Geometry check sheet. Reference: the model listing, model coordinates, mm. A direction names the side the tool comes from. Give positions to 0.01 mm unless a question says otherwise; leave off trailing zeros. Loops run counter-clockwise (first coordinate to the right, second up) from the corner with the lowest first, then second, coordinate; pieces in that order, holes last. Notation, with made-up numbers: (62, 76) -> (94, 76) arc R25 ccw to (94, 114) -> close; hole circle Ø10 at (59, 4.25). An arc over 180 degrees is marked (long way). One line per item, written item: value. Start each with the question number.
(1) Tool access check on faces 4 (the face through (5, -2, 10)), 5 (the face through (-1.73, -7.81, 6.96)). Record the directions out of +Z, -Z, +X, -X, +Y, -Y that give a thin tool (end or side, any length) a straight path to the whole face; none if there is none.
(2) Sectioned sample at A-A, the plane y = 0. Record the cut outline in (x, z).
(3) Draft check along Y on faces 1 (the face through (-14.985, 0.66, 1.986)), 2 (the face through (4.006, 1.262, 4.944)), 3 (the face through (6, -6, 4)). Enter one of: pulls with the +Y half, pulls with the -Y half, needs draft (parallel to the pull), parting line crosses it, or undercut.
(4) Scan lines: line 1 along Y through (x, z) = (-0.25, 8.75); line 2 along Z through (x, y) = (-10.5, 4.75); line 3 along X through (y, z) = (2, 2.5). Record each from-to range of solid material in increasing order. Write a range as from..to.
(5) Gauge pin test, flat ends, axial feed: pin 1 Ø5 at (x, z) = (-9, 9) entering from -Y; pin 2 Ø4 at (x, z) = (-9, 8) entering from -Y; pin 3 Ø9.5 at (x, y) = (0, 0) entering from -Z. Record the tip position at first contact, or that the pin passes through.
(6) Sectioned sample at C-C, the plane z = 2.5. Record the cut outline in (x, y).
from build123d import *

# Parameters (mm, degrees)
CYLINDER_R        = 15
CYLINDER_DEPTH    = 4
CYLINDER002_R     = 8
CYLINDER002_DEPTH = 10
CYLINDER003_R     = 4.2
CYLINDER003_DEPTH = 10
CHAMFER_SIZE      = 1
CHAMFER001_SIZE   = 1


with BuildPart() as part:
    # Cylinder → Cylinder (join)
    with BuildSketch(Plane.XY):
        Circle(CYLINDER_R)
    extrude(amount=CYLINDER_DEPTH)

    # Cylinder002 → Cylinder002 (join)
    with BuildSketch(Plane.XY):
        Circle(CYLINDER002_R)
    extrude(amount=CYLINDER002_DEPTH)

    # Cylinder003 → Cylinder003 (cut)
    with BuildSketch(Plane.XY):
        Circle(CYLINDER003_R)
    extrude(amount=CYLINDER003_DEPTH, mode=Mode.SUBTRACT)

    # Chamfer
    chamfer_edges = [part.edges().sort_by_distance(p)[0] for p in [
        (-15, 0, 4),
        (15, 0, 2),
        (-15, 0, 0),
    ]]
    chamfer(chamfer_edges, length=CHAMFER_SIZE)

    # Chamfer001
    chamfer001_edges = [part.edges().sort_by_distance(p)[0] for p in [
        (-4.2, 0, 10),
        (4.2, 0, 5),
        (-4.2, 0, 0),
    ]]
    chamfer(chamfer001_edges, length=CHAMFER001_SIZE)


solid = part.part
Calculated:
1. face 4: +Z, +X, -X, +Y, -Y
1. face 5: +Z
2. outline: (-15, 1) -> (-14, 0) -> (-5.2, 0) -> (-4.2, 1) -> (-4.2, 9) -> (-5.2, 10) -> (-8, 10) -> (-8, 4) -> (-14, 4) -> (-15, 3) -> close; (4.2, 1) -> (5.2, 0) -> (14, 0) -> (15, 1) -> (15, 3) -> (14, 4) -> (8, 4) -> (8, 10) -> (5.2, 10) -> (4.2, 9) -> close
3. face 1: parting line crosses it
3. face 2: undercut
3. face 3: needs draft
4. line 1: y = -8..-4.19, 4.19..8
4. line 2: z = 0..4
4. line 3: x = -14.87..-3.69, 3.69..14.87
5. pin 1: stops at y = -4.66
5. pin 2: stops at y = -3.87
5. pin 3: stops at z = 0.45
6. outline: circle Ø30 at (0, 0); hole circle Ø8.4 at (0, 0)
